Build history of the part. All positions in model axes, mm. Face numbers are marked on the shaded views. A direction names the side the tool comes from. Round coordinates to 2 decimals unless told otherwise and drop trailing zeros. Write each loop counter-clockwise with the first axis right and the second up, starting at its lowest first coordinate (ties: lowest second). Pieces come first, ordered by that corner, then holes. Notation, with made-up numbers: (4.25, 8.5) - (9.25, 8.5) arc R22 cw to (9.25, 30.5) - close; hole circle Ø5 at (46.25, 55). An arc over 180 degrees is marked (long way). Write each question's results on one line, items separated by ' | '.
from build123d import *

# Parameters (mm, degrees)
SKETCH_1_W          = 57
SKETCH_1_H          = 49
SKETCH_1_W_2        = 53
SKETCH_1_H_2        = 45
EXTRUDE_1_DEPTH     = 5
EXTRUDE_2_DEPTH     = 147
SKETCH_3_W          = 57
SKETCH_3_H          = 49
SKETCH_3_W_2        = 53
SKETCH_3_H_2        = 45
EXTRUDE_3_DEPTH     = 8
SKETCH_5_W          = 57
SKETCH_5_H          = 49
EXTRUDE_4_DEPTH     = 1
SKETCH_7_W          = 57
SKETCH_7_H          = 49
EXTRUDE_6_DEPTH     = 1
SKETCH_8_W          = 1.8
SKETCH_8_H          = 3
SKETCH_8_W_2        = 0.5
SKETCH_8_H_2        = 1.5
CUT_EXTRUDE_1_DEPTH = 2
SKETCH_9_W          = 2.6
SKETCH_9_H          = 10
EXTRUDE_7_DEPTH     = 4
SKETCH_10_W         = 57
SKETCH_10_H         = 49
EXTRUDE_8_DEPTH     = 1
SKETCH_11_R         = 2
CUT_EXTRUDE_2_DEPTH = 6
FILLET_2_R          = 5


with BuildPart() as part:
    # Эскиз1 → Бобышка-Вытянуть1 (new body)
    with BuildSketch(Plane(origin=(0, 0, 0), x_dir=(0, 0, -1), z_dir=(1, 0, 0))):
        Rectangle(SKETCH_1_W, SKETCH_1_H)
        Rectangle(SKETCH_1_W_2, SKETCH_1_H_2, mode=Mode.SUBTRACT)
    extrude(amount=-EXTRUDE_1_DEPTH)

    # Эскиз2 → Бобышка-Вытянуть2 (add)
    with BuildSketch(Plane(origin=(-5, 0, 0), x_dir=(0, 0, -1), z_dir=(1, 0, 0))):
        Polygon((-28.5, 24.5), (-21.5, 24.5), (-21.5, 22.5), (-26.5, 22.5), (-26.5, 17.5), (-28.5, 17.5), align=None)
        Polygon((-28.5, -24.5), (-28.5, -17.5), (-26.5, -17.5), (-26.5, -22.5), (-21.5, -22.5), (-21.5, -24.5), align=None)
        Polygon((28.5, 24.5), (21.5, 24.5), (21.5, 22.5), (26.5, 22.5), (26.5, 17.5), (28.5, 17.5), align=None)
        Polygon((26.5, -22.5), (21.5, -22.5), (21.5, -24.5), (28.5, -24.5), (28.5, -17.5), (26.5, -17.5), align=None)
    extrude(amount=-EXTRUDE_2_DEPTH)

    # Эскиз3 → Бобышка-Вытянуть3 (add)
    with BuildSketch(Plane(origin=(-152, 0, 0), x_dir=(0, 0, -1), z_dir=(1, 0, 0))):
        Rectangle(SKETCH_3_W, SKETCH_3_H)
        Rectangle(SKETCH_3_W_2, SKETCH_3_H_2, mode=Mode.SUBTRACT)
    extrude(amount=-EXTRUDE_3_DEPTH)

    # Эскиз5 → Бобышка-Вытянуть4 (add)
    with BuildSketch(Plane(origin=(0, 0, 0), x_dir=(0, 0, -1), z_dir=(1, 0, 0))):
        Rectangle(SKETCH_5_W, SKETCH_5_H)
    extrude(amount=EXTRUDE_4_DEPTH)

    # Эскиз7 → Бобышка-Вытянуть6 (add)
    with BuildSketch(Plane.ZY.offset(160)):
        Rectangle(SKETCH_7_W, SKETCH_7_H)
    extrude(amount=EXTRUDE_6_DEPTH)

    # Эскиз8 → Вырез-Вытянуть1 (cut)
    with BuildSketch(Plane.ZY.offset(161)):
        with Locations((21.6, -23)):
            Rectangle(SKETCH_8_W, SKETCH_8_H)
        with Locations((17.8, -23)):
            Rectangle(SKETCH_8_W, SKETCH_8_H)
        with Locations((14.65, -23.75)):
            Rectangle(SKETCH_8_W_2, SKETCH_8_H_2)
        with Locations((13.15, -23.75)):
            Rectangle(SKETCH_8_W_2, SKETCH_8_H_2)
        with Locations((11.65, -23.75)):
            Rectangle(SKETCH_8_W_2, SKETCH_8_H_2)
        with Locations((10.15, -23.75)):
            Rectangle(SKETCH_8_W_2, SKETCH_8_H_2)
        with Locations((8.65, -23.75)):
            Rectangle(SKETCH_8_W_2, SKETCH_8_H_2)
        with Locations((7.15, -23.75)):
            Rectangle(SKETCH_8_W_2, SKETCH_8_H_2)
        with Locations((5.65, -23.75)):
            Rectangle(SKETCH_8_W_2, SKETCH_8_H_2)
    extrude(amount=-CUT_EXTRUDE_1_DEPTH, mode=Mode.SUBTRACT)

    # Эскиз9 → Бобышка-Вытянуть7 (add)
    with BuildSketch(Plane(origin=(1, 0, 0), x_dir=(0, 0, -1), z_dir=(1, 0, 0))):
        Polygon((24.5, -20.5), (-24.5, -20.5), (-24.5, -18.5), (-28.5, -18.5), (-28.5, -24.5), (28.5, -24.5), (28.5, 8.5), (24.5, 8.5), align=None)
        Polygon((24.5, 20.5), (-24.5, 20.5), (-24.5, -8.5), (-28.5, -8.5), (-28.5, 24.5), (28.5, 24.5), (28.5, 18.5), (24.5, 18.5), align=None)
        with Locations((0, -13.5)):
            Rectangle(SKETCH_9_W, SKETCH_9_H)
        with Locations((0, 13.5)):
            Rectangle(SKETCH_9_W, SKETCH_9_H)
    extrude(amount=EXTRUDE_7_DEPTH)

    # Эскиз10 → Бобышка-Вытянуть8 (add)
    with BuildSketch(Plane(origin=(5, 0, 0), x_dir=(0, 0, -1), z_dir=(1, 0, 0))):
        Rectangle(SKETCH_10_W, SKETCH_10_H)
    extrude(amount=EXTRUDE_8_DEPTH)

    # Эскиз11 → Вырез-Вытянуть2 (cut)
    with BuildSketch(Plane(origin=(6, 0, 0), x_dir=(0, 0, -1), z_dir=(1, 0, 0))):
        Circle(SKETCH_11_R)
    extrude(amount=-CUT_EXTRUDE_2_DEPTH, mode=Mode.SUBTRACT)

    # Скругление2
    fillet_2_edges = [part.edges().sort_by_distance(p)[0] for p in [
        (-77.5, 24.5, 28.5),
        (-77.5, 24.5, -28.5),
        (-77.5, -24.5, -28.5),
        (-77.5, -24.5, 28.5),
    ]]
    fillet(fillet_2_edges, radius=FILLET_2_R)


solid = part.part
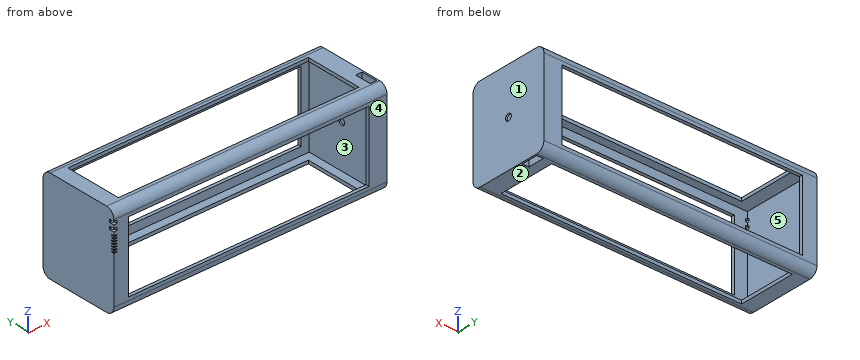
(1) Drill centre lines: probe 1 along X at (y, z) = (3, -8.5); probe 2 along Z at (x, y) = (-88, -19); probe 3 along Y at (x, z) = (5.6, 0). Where is each one in solid material? Low to high. Write a range as [from, to].
Worked answers:
probe 1: x = [-161, -160], [0, 1], [5, 6] | probe 2: z = [-28.5, -26.5], [26.5, 28.5] | probe 3: y = [-24.5, -2], [2, 24.5]
(2) Slice it at C-C, the plane x = -57.5. Write the cut outline in (y, z), and give its area (3 significant figures).
Worked answers:
outline: (-24.5, -23.5) arc R5 ccw to (-19.5, -28.5) - (-17.5, -28.5) - (-17.5, -26.5) - (-22.5, -26.5) - (-22.5, -21.5) - (-24.5, -21.5) - close; (-24.5, 21.5) - (-22.5, 21.5) - (-22.5, 26.5) - (-17.5, 26.5) - (-17.5, 28.5) - (-19.5, 28.5) arc R5 ccw to (-24.5, 23.5) - close; (17.5, -28.5) - (19.5, -28.5) arc R5 ccw to (24.5, -23.5) - (24.5, -21.5) - (22.5, -21.5) - (22.5, -26.5) - (17.5, -26.5) - close; (17.5, 26.5) - (22.5, 26.5) - (22.5, 21.5) - (24.5, 21.5) - (24.5, 23.5) arc R5 ccw to (19.5, 28.5) - (17.5, 28.5) - close | area: 74.5 mm2
(3) Slice it at B-B, the plane y = 4.5. Write the cut outline in (x, z).
Worked answers:
outline: (-161, -28.5) - (-152, -28.5) - (-152, -26.5) - (-160, -26.5) - (-160, 26.5) - (-152, 26.5) - (-152, 28.5) - (-161, 28.5) - close; (-5, -28.5) - (6, -28.5) - (6, 28.5) - (-5, 28.5) - (-5, 26.5) - (0, 26.5) - (0, -26.5) - (-5, -26.5) - close; hole (1, -24.5) - (5, -24.5) - (5, 24.5) - (1, 24.5) - close
(4) Tool access for the marked faces 4 and 5: list every direction of +Z, -Z, +X, -X, +Y, -Y with a clear straight run to the whole face (end or side of a thin tool).
Worked answers:
face 4: +Z, -Z, +X, -X, -Y | face 5: none
(5) Two-plate mould, pull along Z, no slides. Class the marked faces 1, 2 and 3: released by +Z, released by -Z, zero draft, split by the parting line, or undercut.
Worked answers:
face 1: zero draft | face 2: released by -Z | face 3: undercut
(6) Flat gauge pins, fed straight in: pin 1 Ø1.6 at (x, y) = (-160.5, -23.5) entering from -Z; pin 2 Ø1 at (x, z) = (-91, -27) entering from +Y; pin 3 Ø2 at (x, z) = (2.5, -26) entering from -Y. Where does each tip first touch, or does it go through?
Worked answers:
pin 1: stops at z = -27.34 | pin 2: stops at y = 23.5 | pin 3: stops at y = -24.27
(7) Slice it at A-A, the plane z = -6. Write the cut outline in (x, y), and give its area (3 significant figures).
Worked answers:
outline: (-161, -24.5) - (-152, -24.5) - (-152, -22.5) - (-160, -22.5) - (-160, 22.5) - (-152, 22.5) - (-152, 24.5) - (-161, 24.5) - close; (-5, -24.5) - (6, -24.5) - (6, 24.5) - (-5, 24.5) - (-5, 22.5) - (0, 22.5) - (0, -22.5) - (-5, -22.5) - close; hole (1, -20.5) - (5, -20.5) - (5, 20.5) - (1, 20.5) - close | area: 231 mm2
